Part model, mm, in its own coordinate system. Face numbers are marked on the shaded views. Coordinates: 2 decimals unless noted, no trailing zeros. Order: outer loops, then holes, each group sorted by start corner. A loop starts at its lowest first (then second) coordinate and runs counter-clockwise, first axis right, second up.
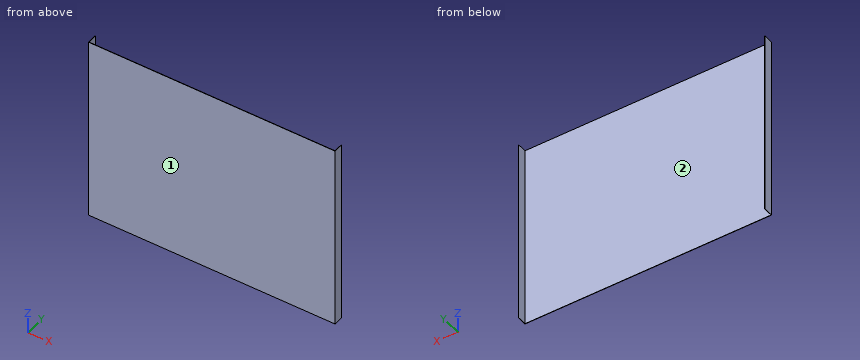
Autodesk Inventor part; units mm, degrees
ref_plane "YZ Plane" through (0, 0, 0) normal (1, 0, 0) x (0, 1, 0)
ref_plane "XZ Plane" through (0, 0, 0) normal (0, 1, 0) x (-1, 0, 0)
ref_plane "XY Plane" through (0, 0, 0) normal (0, 0, 1) x (1, 0, 0)
sketch "Эскиз1" plane through (0, 0, 0) normal (0, 1, 0) x (-1, 0, 0)
  line L0 (13.83, 15.6551) -> (-786.17, 15.6551)
  line L1 (-786.17, 15.6551) -> (-786.17, -584.3449)
  line L2 (-786.17, -584.3449) -> (13.83, -584.3449)
  line L3 (13.83, -584.3449) -> (13.83, 15.6551)
  point P0 (0, 0)
  dimension "d0" = 800
  dimension "d1" = 600
extrude "Выдавливание1" add sketch "Эскиз1" along normal blind 1
sketch "Эскиз2" plane through (0, 1, 0) normal (0, 1, 0) x (1, 0, 0)
  point P0 (0, 0)
sketch "Эскиз3" plane through (0, 1, 0) normal (0, 1, 0) x (1, 0, 0)
  line L0 (-13.83, 584.3449) -> (-13.83, -15.6551)
  line L1 (-13.83, -15.6551) -> (-12.83, -15.6551)
  line L2 (-12.83, -15.6551) -> (-12.83, 584.3449)
  line L3 (-12.83, 584.3449) -> (-13.83, 584.3449)
  line L4 (-13.83, 584.3449) -> (-13.83, -15.6551)
  line L5 (-13.83, -15.6551) -> (786.17, -15.6551)
  line L6 (786.17, -15.6551) -> (785.17, -15.6551)
  line L7 (785.17, -15.6551) -> (785.17, 584.3449)
  line L8 (785.17, 584.3449) -> (786.17, 584.3449)
  line L9 (786.17, 584.3449) -> (786.17, -15.6551)
  point P0 (0, 0)
  dimension "d4" = 1
  dimension "d5" = 600
  dimension "d6" = 1
  dimension "d7" = 600
extrude "Выдавливание2" add sketch "Эскиз3" along normal blind 30 contours L3 L2 L1 L0
sketch "Эскиз4" plane through (0, 1, 0) normal (0, 1, 0) x (1, 0, 0)
  line L0 (786.17, -15.6551) -> (785.17, -15.6551)
  line L1 (785.17, -15.6551) -> (785.17, 584.3449)
  line L2 (785.17, 584.3449) -> (786.17, 584.3449)
  line L3 (786.17, 584.3449) -> (786.17, -15.6551)
  point P0 (0, 0)
  dimension "d10" = 1
  dimension "d11" = 600
extrude "Выдавливание3" add sketch "Эскиз4" along normal blind 30
properties part number "Полка"
(1) Slice it at A-A, the plane y = 26. Give the cut face in (x, z), then the cut area to 3 significant figures.
(2) Slice it at C-C, the plane x = 334. Give the cut face in (y, z).
(3) Slice it at B-B, the plane z = -309.5. Give the cut face in (x, y), then the cut area to 3 significant figures.
(4) Probe line 1 (X direction, y = 24.5, z = -209.5); line 2 (Y direction, x = 615.5, z = -53). List the from-to ranges inside material, lowest first.
(5) Drop flat-ended pins along their axis: pin 1 (1 mm diameter, centred on x = 386.5, z = -445.5, fed in from +Y); pin 2 (10 mm diameter, centred on x = 229.5, y = 6.5, fed in from +Z). Give the stop position or say it passes through.
(6) Pull direction X, two halves, no side cores. Call the marked faces 1 and 2: +X half, -X half, draft (parallel to the pull), parting line (faces both ways), or undercut.
Here are the results:
1. outline: (-13.83, -584.34) - (-12.83, -584.34) - (-12.83, 15.66) - (-13.83, 15.66) - close; (785.17, -584.34) - (786.17, -584.34) - (786.17, 15.66) - (785.17, 15.66) - close
1. area: 1,200 mm2
2. outline: (0, -584.34) - (1, -584.34) - (1, 15.66) - (0, 15.66) - close
3. outline: (-13.83, 0) - (786.17, 0) - (786.17, 31) - (785.17, 31) - (785.17, 1) - (-12.83, 1) - (-12.83, 31) - (-13.83, 31) - close
3. area: 860 mm2
4. line 1: x = -13.83 to -12.83, 785.17 to 786.17
4. line 2: y = 0 to 1
5. pin 1: stops at y = 1
5. pin 2: passes through
6. face 1: draft
6. face 2: undercut
